Source: CAD feature listing. Evaluate the final solid. Frame: model axes, mm. Give positions to 0.01 mm unless a question says otherwise; leave off trailing zeros. Loops run counter-clockwise (first coordinate to the right, second up) from the corner with the lowest first, then second, coordinate; pieces in that order, holes last. Notation, with made-up numbers: (-38, -23.75) - (14, -23.75) arc R19 ccw to (14, -6.75) - close; hole circle Ø4 at (73.5, 76). An arc over 180 degrees is marked (long way). Write each question's results on one line, items separated by ' | '. Start each with the question number.
(1) Cut plane C-C on z = 1. Return the cut outline in (x, y).
(2) Contact query for flat-ended pins moving along their axis: pin 1 (1.5 mm diameter, centred on y = 1.5, z = 65, fed in from -X); pin 2 (0.9 mm diameter, centred on x = 62, y = 2, fed in from +Z); pin 3 (1.5 mm diameter, centred on y = 1.5, z = 54.5, fed in from +X); pin 4 (3 mm diameter, centred on x = 40.36, z = 74.54, fed in from -Y). Output: stop coordinate, or through.
(3) Material intervals for line 1 along X through (y, z) = (1.9, -75); line 2 along X through (y, z) = (5.5, -18), sorted ascending. Write a range as [from, to].
(4) Cut plane A-A on y = 4.5. Give the number of separate pieces and of enclosed holes in the cut face, then the cut area to 3 significant figures.
(5) Cut plane B-B on x = -47. Return the cut outline in (y, z).
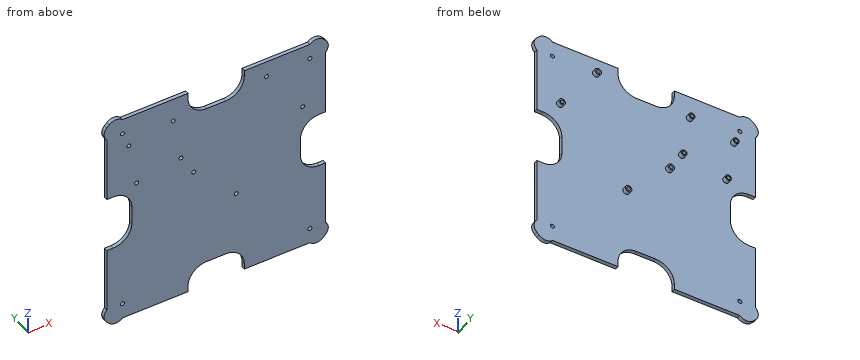
from build123d import *

# Parameters (mm, degrees)
SHELL_BOSS_DEPTH             = 3
SHELL_FILET_R                = 7.5
SHELL_PILLAR_HOLE_DEPTH      = 127.973590966
SHELL_PILLAR_HOLE_DEPTH_BACK = 127.973590966
SKETCH5_R                    = 1.6
SKETCH16_R                   = 2.625
ARDUINO_MOUNT_BOSS_DEPTH     = 3.25
SKETCH22_R                   = 1.55
ARDUINO_CUT_DEPTH            = 6.25
SKETCH20_R                   = 2.4
BOSS_EXTRUDE9_DEPTH          = 3.5
SKETCH37_R                   = 1.55
CUT_EXTRUDE4_DEPTH           = 6.5
CUT_EXTRUDE5_DEPTH           = 128.104456266
CUT_EXTRUDE5_DEPTH_BACK      = 128.104456266
SKETCH38_W                   = 45
SKETCH38_H                   = 20
SKETCH38_W_2                 = 20
SKETCH38_H_2                 = 45
FILLET1_R                    = 15


with BuildPart() as part:
    # Sketch1 → shell-boss (new body)
    with BuildSketch(Plane(origin=(0, 0, 0), x_dir=(1, 0, 0), z_dir=(0, 1, 0))):
        with BuildLine():
            Line((87.5, 75), (96.856853139, 75))
            ThreePointArc((96.856853139, 75), (86.620580695, 86.620580695), (75, 96.856853139))
            Line((75, 96.856853139), (75, 87.5))
            Line((75, 87.5), (-75, 87.5))
            Line((-75, 87.5), (-75, 96.856853139))
            ThreePointArc((-75, 96.856853139), (-86.620580695, 86.620580695), (-96.856853139, 75))
            Line((-96.856853139, 75), (-87.5, 75))
            Line((-87.5, 75), (-87.5, -75))
            Line((-87.5, -75), (-96.856853139, -75))
            ThreePointArc((-96.856853139, -75), (-86.620580695, -86.620580695), (-75, -96.856853139))
            Line((-75, -96.856853139), (-75, -87.5))
            Line((-75, -87.5), (75, -87.5))
            Line((75, -87.5), (75, -96.856853139))
            ThreePointArc((75, -96.856853139), (86.620580695, -86.620580695), (96.856853139, -75))
            Line((96.856853139, -75), (87.5, -75))
            Line((87.5, -75), (87.5, 75))
        make_face()
    extrude(amount=SHELL_BOSS_DEPTH)

    # shell-filet
    # the kernel refuses this fillet: 7.5 mm, written as the material it takes off along each edge
    with BuildSketch(Plane(origin=(-96.856853139, -35.154925645, 75), x_dir=(1, 0, 0), z_dir=(0, 1, 0)), Plane(origin=(-75, -35.154925645, -96.856853139), x_dir=(0, 0, 1), z_dir=(0, 1, 0)), Plane(origin=(96.856853139, -35.154925645, -75), x_dir=(-1, 0, 0), z_dir=(0, 1, 0))) as shell_filet_piece_1:
        with BuildLine():
            CenterArc((14.59802961, -5.364705882), SHELL_FILET_R, 134.332691644, 90)
            Line((9.233323727, -10.605882353), (9.12602961, -10.710705882))
            ThreePointArc((9.12602961, -10.710705882), (4.351219382, -5.53403146), (-0.118600228, -0.091836735))
            Line((-0.118600228, -0.091836735), (0, 0.15))
            ThreePointArc((0, 0.15), (4.67842657, 0.15), (9.25202961, 0.107294118))
            Line((9.25202961, 0.107294118), (9.356853139, 0))
        make_face()
    extrude(amount=73.30985129, mode=Mode.SUBTRACT)
    with BuildSketch(Plane(origin=(-96.856853139, -35.154925645, -75), x_dir=(0.656616644600313, 0, -0.7542244904760296), z_dir=(0, 1, 0)), Plane(origin=(75, -35.154925645, -96.856853139), x_dir=(0.7542244904760282, 0, 0.6566166446003142), z_dir=(0, 1, 0)), Plane(origin=(96.856853139, -35.154925645, 75), x_dir=(-0.656616644600296, 0, 0.7542244904760443), z_dir=(0, 1, 0)), Plane(origin=(-75, -35.154925645, 96.856853139), x_dir=(-0.7542244904760502, 0, -0.6566166446002892), z_dir=(0, 1, 0))) as shell_filet_piece_2:
        with BuildLine():
            CenterArc((13.631501781, -7.487636269), SHELL_FILET_R, 86.709654831, 90)
            Line((6.143865512, -7.057167791), (5.994112787, -7.048558422))
            ThreePointArc((5.994112787, -7.048558422), (2.958799083, -3.627076392), (-0.113133674, -0.098492497))
            Line((-0.113133674, -0.098492497), (-0.00860937, 0.149752725))
            ThreePointArc((-0.00860937, 0.149752725), (7.030985129, 0.351940947), (14.070579628, 0.149752725))
            Line((14.070579628, 0.149752725), (14.061970258, 0))
        make_face()
    extrude(amount=73.30985129, mode=Mode.SUBTRACT)
    with BuildSketch(Plane(origin=(75, -35.154925645, 96.856853139), x_dir=(0.754224490476002, 0, -0.6566166446003444), z_dir=(0, 1, 0))) as shell_filet_piece_3:
        with BuildLine():
            CenterArc((13.631501781, 7.487636269), SHELL_FILET_R, 183.290345169, 90)
            Line((6.143865512, 7.057167791), (5.994112787, 7.048558422))
            ThreePointArc((5.994112787, 7.048558422), (2.958799083, 3.627076392), (-0.113133674, 0.098492497))
            Line((-0.113133674, 0.098492497), (-0.00860937, -0.149752725))
            ThreePointArc((-0.00860937, -0.149752725), (7.030985129, -0.351940947), (14.070579628, -0.149752725))
            Line((14.070579628, -0.149752725), (14.061970258, 0))
        make_face()
    extrude(amount=73.30985129, mode=Mode.SUBTRACT)

    # Sketch5 → shell-pillar-hole (cut, two sides: drawn at the far end of the back side and taken through both)
    with BuildSketch(Plane(origin=(0, 3, 0), x_dir=(1, 0, 0), z_dir=(0, 1, 0)).offset(-SHELL_PILLAR_HOLE_DEPTH_BACK)):
        with Locations(Location((75, -75, 0), (0, 0, 270))):
            Circle(SKETCH5_R)
        with Locations(Location((-75, -75, 0), (0, 0, 270))):
            Circle(SKETCH5_R)
        with Locations(Location((75, 75, 0), (0, 0, 270))):
            Circle(SKETCH5_R)
        with Locations(Location((-75, 75, 0), (0, 0, 270))):
            Circle(SKETCH5_R)
    extrude(amount=SHELL_PILLAR_HOLE_DEPTH + SHELL_PILLAR_HOLE_DEPTH_BACK, mode=Mode.SUBTRACT)

    # Sketch16 → arduino-mount-boss (add)
    with BuildSketch(Plane(origin=(0, 3, 0), x_dir=(1, 0, 0), z_dir=(0, 1, 0))):
        with Locations(Location((16.113832172, 18.065022624, 0), (0, 0, 90))):
            Circle(SKETCH16_R)
        with Locations(Location((-18.065022624, -16.113832172, 0), (0, 0, 90))):
            Circle(SKETCH16_R)
        with Locations(Location((69.241027385, -35.062172588, 0), (0, 0, 90))):
            Circle(SKETCH16_R)
        with Locations(Location((40.360523699, -74.539378496, 0), (0, 0, 90))):
            Circle(SKETCH16_R)
    extrude(amount=ARDUINO_MOUNT_BOSS_DEPTH)

    # Sketch22 → arduino-cut (cut)
    with BuildSketch(Plane(origin=(0, 6.25, 0), x_dir=(1, 0, 0), z_dir=(0, 1, 0))):
        with Locations(Location((16.113832172, 18.065022624, 0), (0, 0, 270))):
            Circle(SKETCH22_R)
        with Locations(Location((-18.065022624, -16.113832172, 0), (0, 0, 270))):
            Circle(SKETCH22_R)
        with Locations(Location((69.241027385, -35.062172588, 0), (0, 0, 270))):
            Circle(SKETCH22_R)
        with Locations(Location((40.360523699, -74.539378496, 0), (0, 0, 270))):
            Circle(SKETCH22_R)
    extrude(amount=-ARDUINO_CUT_DEPTH, mode=Mode.SUBTRACT)

    # Sketch20 → Boss-Extrude9 (add)
    with BuildSketch(Plane(origin=(0, 3, 0), x_dir=(1, 0, 0), z_dir=(0, 1, 0))):
        with Locations(Location((-63.655367651, -26.687870454, 0), (0, 0, 270))):
            Circle(SKETCH20_R)
        with Locations(Location((-28.202288543, -32.93920485, 0), (0, 0, 270))):
            Circle(SKETCH20_R)
        with Locations(Location((-34.453622939, -68.392283958, 0), (0, 0, 270))):
            Circle(SKETCH20_R)
        with Locations(Location((-69.906702047, -62.140949562, 0), (0, 0, 270))):
            Circle(SKETCH20_R)
    extrude(amount=BOSS_EXTRUDE9_DEPTH)

    # Sketch37 → Cut-Extrude4 (cut)
    with BuildSketch(Plane(origin=(0, 6.5, 0), x_dir=(1, 0, 0), z_dir=(0, 1, 0))):
        with Locations(Location((-63.655367651, -26.687870454, 0), (0, 0, 270))):
            Circle(SKETCH37_R)
        with Locations(Location((-28.202288543, -32.93920485, 0), (0, 0, 270))):
            Circle(SKETCH37_R)
        with Locations(Location((-69.906702047, -62.140949562, 0), (0, 0, 270))):
            Circle(SKETCH37_R)
        with Locations(Location((-34.453622939, -68.392283958, 0), (0, 0, 270))):
            Circle(SKETCH37_R)
    extrude(amount=-CUT_EXTRUDE4_DEPTH, mode=Mode.SUBTRACT)

    # Sketch38 → Cut-Extrude5 (cut, two sides: drawn at the far end of the back side and taken through both)
    with BuildSketch(Plane.XZ.offset(-CUT_EXTRUDE5_DEPTH_BACK)):
        with Locations((0, 77.5)):
            Rectangle(SKETCH38_W, SKETCH38_H)
        with Locations((77.5, 0)):
            Rectangle(SKETCH38_W_2, SKETCH38_H_2)
        with Locations((0, -77.5)):
            Rectangle(SKETCH38_W, SKETCH38_H)
        with Locations((-77.5, 0)):
            Rectangle(SKETCH38_W_2, SKETCH38_H_2)
    extrude(amount=CUT_EXTRUDE5_DEPTH + CUT_EXTRUDE5_DEPTH_BACK, mode=Mode.SUBTRACT)

    # Fillet1
    fillet1_edges = [part.edges().sort_by_distance(p)[0] for p in [
        (22.5, 1.5, 67.5),
        (-22.5, 1.5, 67.5),
        (67.5, 1.5, -22.5),
        (67.5, 1.5, 22.5),
        (-22.5, 1.5, -67.5),
        (22.5, 1.5, -67.5),
        (-67.5, 1.5, 22.5),
        (-67.5, 1.5, -22.5),
    ]]
    fillet(fillet1_edges, radius=FILLET1_R)


solid = part.part
Ans:
1) outline: (-67.5, 0) - (67.5, 0) - (67.5, 3) - (-67.5, 3) - close
2) pin 1: x = -87.5 | pin 2: z = 87.5 | pin 3: x = 87.5 | pin 4: through
3) line 1: [-87.5, -76.6], [-73.4, -20.49], [20.49, 73.4], [76.6, 87.5] | line 2: [13.49, 14.57], [17.66, 18.74]
4) separate pieces: 8 | enclosed holes: 8 | area: 98.6 mm^2
5) outline: (0, -87.5) - (3, -87.5) - (3, 87.5) - (0, 87.5) - close
